Check sheet for the modelled part. Datum: model origin and axes. Units: mm. Face numbers are marked on the shaded views. A direction names the side the tool comes from. Give positions to 0.01 mm unless a question says otherwise; leave off trailing zeros. Order: outer loops, then holes, each group sorted by start corner. A loop starts at its lowest first (then second) coordinate and runs counter-clockwise, first axis right, second up. Notation, with made-up numbers: (22.5, 50.25) -> (63.5, 50.25) arc R16 ccw to (63.5, 72.25) -> close; hole circle Ø1 at (-27, 11). An arc over 180 degrees is marked (long way). Write each question's results on one line, items separated by ' | '.
from build123d import *

# Parameters (mm, degrees)
F0_R     = 4.5
F1_DEPTH = 6
F2_T     = -2
F3_R     = 2
F4_DEPTH = 5
F5_T     = 1
F6_R     = 1
F7_DEPTH = 12.5


# Not quite as in the source:
# - a shell that OpenCascade refuses in one call is made with other operations: the cavity is built on its own and cut out


with BuildPart() as f1:
    # F0 (on Top) → F1 (new body)
    with BuildSketch(Plane.XY):
        Circle(F0_R)
    extrude(amount=F1_DEPTH)

    # F2
    f2_openings = [f1.faces().sort_by_distance(p)[0] for p in [
        (0, 0, 6),
    ]]
    offset(amount=F2_T, openings=f2_openings)

    # F3 (on face) → F4 (join)
    with BuildSketch(Plane(origin=(0, 0, 0), x_dir=(1, 0, 0), z_dir=(0, 0, -1))):
        Circle(F3_R)
    extrude(amount=F4_DEPTH)

    # F5: shell of thickness 1, made by hand


with BuildPart() as f5_core1:
    # F5_t2: copy of F1
    add(f1.part)

    # the walls: a layer under each face that stays
    f5_faces = [f5_core1.faces().sort_by_distance(p)[0] for p in [
        (-4.5, 0, 3),
        (-3, -3, 0),
        (-3, -3, 6),
        (-2, 0, -2.5),
        (-2.5, 0, 4),
        (0, 0, 2),
    ]]
    thicken(f5_faces, amount=-F5_T, mode=Mode.SUBTRACT)

    # F5_s3 → F5_t4 (revolve, cut)
    with BuildSketch(Plane.XZ):
        Polygon((2.01, -0.01), (2, 1), (1, 1), (1, 0), align=None)
    revolve(axis=Axis((0, 0, 0), (0, 0, -1)), mode=Mode.SUBTRACT)

    # F5_s5 → F5_t6 (revolve, cut)
    with BuildSketch(Plane.XZ):
        Polygon((2.49, 2.01), (3.5, 2), (3.5, 1), (2.5, 1), align=None)
    revolve(axis=Axis((0, 0, 2), (0, 0, -1)), mode=Mode.SUBTRACT)


with BuildPart() as f1_1:
    add(f1.part)

    # what is left inside the walls is the cavity
    f5_cavity = [f5_core1.part.solids().sort_by_distance(p)[0] for p in [
        (-0.99, 0, -1),
    ]]
    add(f5_cavity, mode=Mode.SUBTRACT)

    # F6 (on face) → F7 (cut, symmetric)
    with BuildSketch(Plane(origin=(0, 0, 0), x_dir=(1, 0, 0), z_dir=(0, 0, -1))):
        Circle(F6_R)
    extrude(amount=F7_DEPTH, both=True, mode=Mode.SUBTRACT)


solid = f1_1.part
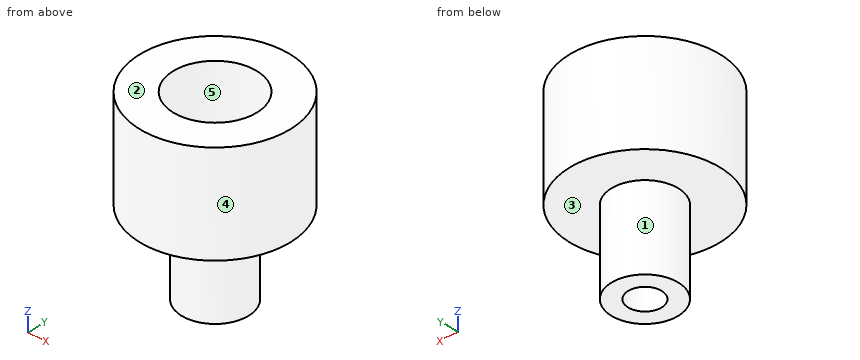
1. Section check D-D on x = 2.25. Record the cut outline in (y, z).
Verdict:
outline: (-3.9, 0) -> (3.9, 0) -> (3.9, 6) -> (1.09, 6) -> (1.09, 2) -> (-1.09, 2) -> (-1.09, 6) -> (-3.9, 6) -> close
2. Gauge pin test, flat ends, axial feed: pin 1 Ø4 at (y, z) = (1, -3.5) entering from -X; pin 2 Ø1.5 at (y, z) = (1.5, 4.5) entering from -X; pin 3 Ø1.5 at (x, y) = (3, 0.5) entering from -Z. Record the tip position at first contact, or that the pin passes through.
Verdict:
pin 1: stops at x = -2 | pin 2: stops at x = -4.44 | pin 3: stops at z = 0
3. Mould release check, pull along X, two halves, no side actions. Record for the marked faces 3, 4 and 5: +X half, -X half, draft (parallel to the pull), parting line (faces both ways), or undercut.
Verdict:
face 3: draft | face 4: parting line | face 5: undercut
4. Access from +Z, -Z, +X, -X, +Y, -Y to the whole of each face (thin tool, end or side, straight path). Record for the marked faces 1 and 2.
Verdict:
face 1: -Z | face 2: +Z, +X, -X, +Y, -Y
5. Section check C-C on z = 1.5. Record the cut outline in (x, y).
Verdict:
outline: circle Ø9 at (0, 0); hole circle Ø2 at (0, 0)
6. Section check A-A on y = 0. Record the cut outline in (x, z).
Verdict:
outline: (-4.5, 0) -> (-2, 0) -> (-2, -5) -> (-1, -5) -> (-1, 2) -> (-2.5, 2) -> (-2.5, 6) -> (-4.5, 6) -> close; (1, -5) -> (2, -5) -> (2, 0) -> (4.5, 0) -> (4.5, 6) -> (2.5, 6) -> (2.5, 2) -> (1, 2) -> close
7. Material ranges on probe 1 along Y at (x, z) = (0, 5.1); probe 2 along X at (y, z) = (0, -1); probe 3 along Y at (x, z) = (0, 0.5), recorded low to high. Write a range as from..to.
Verdict:
probe 1: y = -4.5..-2.5, 2.5..4.5 | probe 2: x = -2..-1, 1..2 | probe 3: y = -4.5..-1, 1..4.5
